Input: part model. Units: mm. Frame: model coordinates. Face numbers are marked on the shaded views. A direction names the side the tool comes from. Coordinates: 2 decimals unless noted, no trailing zeros. Loops run counter-clockwise (first coordinate to the right, second up) from the corner with the lowest first, then second, coordinate; pieces in that order, holes last. Notation, with made-up numbers: (3, -16) -> (61, -16) arc R37 cw to (61, 23) -> close; hole circle Ø9 at (73.25, -33.5). An arc over 180 degrees is marked (long way). Answer as a JSON object with one key per item and string values.
Autodesk Fusion 360 part; units mm, degrees
sketch "Sketch1" plane through (0, 0, 0) normal (0, 0, 1) x (1, 0, 0)
  circle A0 centre (-28, 0) radius 8
  line L0 (0, 0) -> (0, 62.0025)
  circle A1 centre (28, 0) radius 8
  line L1 (-28, 18) -> (28, 18)
  line L2 (-28, -18) -> (28, -18)
  arc A2 (28, -18) -> (28, 18) centre (28, 0) ccw
  arc A3 (-28, 18) -> (-28, -18) centre (-28, 0) ccw
  dimension "d1" = 16
  dimension "d2" = 36
  dimension "d3" = 28
extrude "Extrude1" add sketch "Sketch1" along normal blind 8
sketch "Sketch2" plane through (0, 0, 8) normal (0, 0, 1) x (-1, 0, 0)
  circle A0 centre (28, 0) radius 8
  circle A1 centre (-28, 0) radius 8
  arc A2 (28, -18) -> (28, 18) centre (28, 0) ccw
  line L0 (28, 18) -> (-28, 18)
  arc A3 (-28, 18) -> (-28, -18) centre (-28, 0) ccw
  line L1 (-28, -18) -> (28, -18)
sketch "Sketch3" plane through (0, 0, 8) normal (0, 0, 1) x (-1, 0, 0)
  line L0 (20, -18) -> (-20, -18)
  line L1 (-20, -18) -> (-20, -8)
  line L2 (-20, -8) -> (20, -8)
  line L3 (20, -8) -> (20, -18)
  dimension "d6" = 40
  dimension "d7" = 10
  dimension "d8" = 20
extrude "Extrude2" add sketch "Sketch3" along normal blind 32
sketch "Sketch4" plane through (0, 0, 40) normal (0, 0, 1) x (-1, 0, 0)
  line L0 (20, -8) -> (-20, -8)
  line L1 (-20, -8) -> (-20, -18)
  line L2 (-20, -18) -> (20, -18)
  line L3 (20, -18) -> (20, -8)
  circle A0 centre (-0.2889, -50) radius 10
  line L4 (14.5242, -52.3607) -> (20, -18)
  line L5 (-15.1389, -52.1159) -> (-20, -18)
  arc A1 (-15.1389, -52.1159) -> (14.5242, -52.3607) centre (-0.2889, -50) ccw
  dimension "d11" = 20
  dimension "d12" = 30
  dimension "d13" = 32
extrude "Extrude3" add sketch "Sketch4" against normal blind 10 contours L2 L4 L5 A1
sketch "Sketch5" plane through (0, 0, 40) normal (0, 0, 1) x (-1, 0, 0)
  circle A0 centre (-0.2889, -50) radius 10
  line L0 (20, -8) -> (-20, -8)
  line L1 (-20, -8) -> (-20, -18)
  line L2 (-20, -18) -> (-15.1389, -52.1159)
  arc A1 (-15.1389, -52.1159) -> (14.5242, -52.3607) centre (-0.2889, -50) ccw
  line L3 (14.5242, -52.3607) -> (20, -18)
  line L4 (20, -18) -> (20, -8)
  circle A2 centre (-0.2889, -50) radius 10
  circle A3 centre (-0.2889, -50) radius 15
  dimension "d16" = 20
  dimension "d17" = 30
extrude "Extrude4" add sketch "Sketch5" along normal blind 10 contours A1 A3
sketch "Sketch6" plane through (0, 0, 0) normal (1, 0, 0) x (0, 1, 0)
  curve L0
  curve L1
  line L2 (8, 40) -> (-18, 8)
  curve L3
  line L4 (-18, 8) -> (8, 8)
  line L5 (8, 40) -> (8, 8)
extrude "Extrude5" add sketch "Sketch6" along normal blind 6 and the other way blind 6
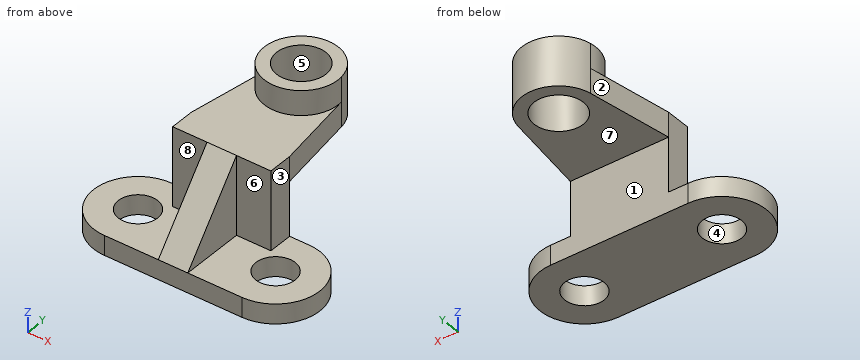
1. Mould query, pull axis X, two halves, no side actions, for the marked faces 1, 2, 3 and 4. Classes: pulls with the +X half, pulls with the -X half, needs draft (parallel to the pull), parting line crosses it, or undercut.
Reply:
{"face 1": "needs draft", "face 2": "pulls with the -X half", "face 3": "pulls with the +X half", "face 4": "undercut"}
2. Pin query (flat end, axial travel): P1, Ø24, axis at x = 4, z = 12.5, coming from the +Y side; P2, Ø11, axis at x = -11, z = 19, coming from the -Y side; P3, Ø5, axis at y = 15, z = 18.5, coming from the +X side; P4, Ø12, axis at x = 0.29, y = 50, coming from the -Z side. Return the tip coordinate at first contact, or that it passes through.
Reply:
{"P1": "stops at y = 18", "P2": "stops at y = -10.92", "P3": "stops at x = 20", "P4": "passes through"}
3. Section query C-C (x = 18). Return loops of the section in (y, z).
Reply:
{"outline": "(-18, 0) -> (18, 0) -> (18, 30) -> (32.04, 30) -> (32.04, 40) -> (8, 40) -> (8, 8) -> (-18, 8) -> close"}
4. Line query: line 1 along Y through (x, z) = (-28, 4.5); line 2 along Z through (x, y) = (6.5, 23); line 3 along Z through (x, y) = (42, -3.5). Output: solid intervals per line, ascending.
Reply:
{"line 1": "y = -18 to -8, 8 to 18", "line 2": "z = 30 to 40", "line 3": "z = 0 to 8"}
5. Section query D-D (z = 22). Return loops of the section in (x, y) (3 decimals), plus the area to 4 significant figures.
Reply:
{"outline": "(-20, 8) -> (-6, 8) -> (-6, -6.625) -> (6, -6.625) -> (6, 8) -> (20, 8) -> (20, 18) -> (-20, 18) -> close", "area": "575.5 mm2"}
6. Access query for the marked faces 5, 6, 7 and 8. Directions: +Z, -Z, +X, -X, +Y, -Y. A direction counts if a zero-diameter tool reaches every point of the face in a straight line with its end or side. Return the directions, or none.
Reply:
{"face 5": "+Z, -Z", "face 6": "+Z, +X, -Y", "face 7": "-Z, +X, -X, +Y", "face 8": "+Z, -X, -Y"}
7. Section query B-B (y = 5). Return loops of the section in (x, z) (3 decimals), plus the area to 3 significant figures.
Reply:
{"outline": "(-45.292, 0) -> (-34.245, 0) -> (-34.245, 8) -> (-45.292, 8) -> close; (-21.755, 0) -> (21.755, 0) -> (21.755, 8) -> (6, 8) -> (6, 36.308) -> (-6, 36.308) -> (-6, 8) -> (-21.755, 8) -> close; (34.245, 0) -> (45.292, 0) -> (45.292, 8) -> (34.245, 8) -> close", "area": "865 mm2"}
8. Section query A-A (y = 44). Return loops of the section in (x, z), plus the area to 3 significant figures.
Reply:
{"outline": "(-15.86, 30) -> (-7.71, 30) -> (-7.71, 50) -> (-13.46, 50) -> (-13.46, 40) -> (-15.86, 40) -> close; (8.29, 30) -> (16.3, 30) -> (16.3, 40) -> (14.04, 40) -> (14.04, 50) -> (8.29, 50) -> close", "area": "276 mm2"}
